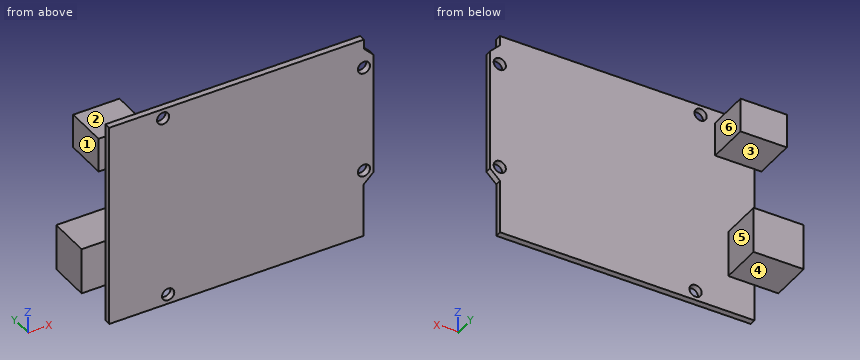
from build123d import *

# Parameters (mm, degrees)
SKETCH1_R           = 1.5875
BOSS_EXTRUDE1_DEPTH = 1.6
SKETCH2_W           = 12
SKETCH2_H           = 8.9
SKETCH2_W_2         = 13
SKETCH2_H_2         = 12
BOSS_EXTRUDE2_DEPTH = 10.9


with BuildPart() as part:
    # Sketch1 → Boss-Extrude1 (new body)
    with BuildSketch(Plane(origin=(0, 0, 0), x_dir=(1, 0, 0), z_dir=(0, 1, 0))):
        Polygon((-34.3, -26.65), (-34.3, 26.65), (31.74, 26.65), (31.74, 12.68), (34.34, 10.18), (34.34, -21.57), (31.8, -24.11), (31.8, -26.65), align=None)
        with Locations(Location((-19, 24.15, 0), (0, 0, 270))):
            Circle(SKETCH1_R, mode=Mode.SUBTRACT)
        with Locations(Location((-20.3, -24.15, 0), (0, 0, 270))):
            Circle(SKETCH1_R, mode=Mode.SUBTRACT)
        with Locations(Location((31.8, 8.91, 0), (0, 0, 270))):
            Circle(SKETCH1_R, mode=Mode.SUBTRACT)
        with Locations(Location((31.8, -19.03, 0), (0, 0, 270))):
            Circle(SKETCH1_R, mode=Mode.SUBTRACT)
    extrude(amount=BOSS_EXTRUDE1_DEPTH)

    # Sketch2 → Boss-Extrude2 (add)
    with BuildSketch(Plane(origin=(0, 1.6, 0), x_dir=(1, 0, 0), z_dir=(0, 1, 0))):
        with Locations((-30.1, -18.9)):
            Rectangle(SKETCH2_W, SKETCH2_H)
        with Locations((-34, 11.05)):
            Rectangle(SKETCH2_W_2, SKETCH2_H_2)
    extrude(amount=BOSS_EXTRUDE2_DEPTH)


solid = part.part
Design review of the part built by this model. Coordinates are the model's own, in mm. Face numbers are marked on the shaded views. A direction names the side the tool comes from. Give positions to 0.01 mm unless a question says otherwise; leave off trailing zeros. Loops run counter-clockwise (first coordinate to the right, second up) from the corner with the lowest first, then second, coordinate; pieces in that order, holes last. Notation, with made-up numbers: M 38.5,-36 L 45.5,-36 A19 cw 45.5,-11 Z; hole C 76,-36 d5. An arc over 180 degrees is marked long. One line per question, with ' | ' between items. Start each with the question number.
1. For the marked faces 4, 5 and 6, list the 3-axis set-ups (+Z, -Z, +X, -X, +Y, -Y) from which the entire face can be reached by the end or side of a thin tool; tool diameter is ignored.
2. Insertion check: P1, Ø8, axis at x = -26, z = -19, coming from the +Y side; P2, Ø1.4, axis at x = -35.5, z = 21, coming from the -Y side; P3, Ø1.9, axis at x = 31.8, z = -8.91, coming from the -Y side; P4, Ø3.5, axis at x = 31.8, z = 19.03, coming from the +Y side. Each pin has a flat end and moves straight along its axis. Give the tip position at first contact, or say it passes through.
3. Add section C-C (z = -24.15). Write out the cut boundary in (x, y).
4. Add section B-B (z = -8.91). Write out the cut boundary in (x, y).
5. To check wall thickness, follow L1, parallel to X at y = 1.05, z = -8.91; L2, parallel to Z at x = -34.5, y = 4.75; L3, parallel to X at y = 0.9, z = -24.15. State the ranges of each line that lie inside material, in increasing order.
6. The part is to be moulded in two halves that separate along Z. For the marked faces 1, 2 and 3, say which applies: released by +Z, released by -Z, zero draft, split by the parting line, or undercut.
7. Add section A-A (y = 2.75). Write out the cut boundary in (x, z), plus the area to 3 significant figures.
8. Add section D-D (x = 27). Write out the cut boundary in (y, z).
Worked out:
1) face 4: -Z, +X, -X, +Y | face 5: -Z, +X, +Y | face 6: +Z, -Z, +X, +Y
2) P1: stops at y = 12.5 | P2: stops at y = 1.6 | P3: passes through | P4: stops at y = 1.6
3) outline: M -34.3,0 L -20.59,0 L -20.59,1.6 L -34.3,1.6 Z; M -17.41,0 L 31.74,0 L 31.74,1.6 L -17.41,1.6 Z
4) outline: M -40.5,1.6 L -34.3,1.6 L -34.3,0 L 30.21,0 L 30.21,1.6 L -27.5,1.6 L -27.5,12.5 L -40.5,12.5 Z; M 33.39,0 L 34.34,0 L 34.34,1.6 L 33.39,1.6 Z
5) L1: x = -34.3 to 30.21, 33.39 to 34.34 | L2: z = -17.05 to -5.05, 14.45 to 23.35 | L3: x = -34.3 to -20.59, -17.41 to 31.74
6) face 1: zero draft | face 2: released by +Z | face 3: undercut
7) outline: M -40.5,-17.05 L -27.5,-17.05 L -27.5,-5.05 L -40.5,-5.05 Z; M -36.1,14.45 L -24.1,14.45 L -24.1,23.35 L -36.1,23.35 Z | area: 263 mm²
8) outline: M 0,-26.65 L 1.6,-26.65 L 1.6,26.65 L 0,26.65 Z
